Build history of the part. All positions in model axes, mm. A direction names the side the tool comes from. Give positions to 0.01 mm unless a question says otherwise; leave off trailing zeros. Loops run counter-clockwise (first coordinate to the right, second up) from the corner with the lowest first, then second, coordinate; pieces in that order, holes last.
1) 3-axis set-ups, long thin cutter, end or side, ignore diameter. For faces 5 (the cylindrical face through (50.56, -3.01, 47.15)), 6 (the flat face through (49, -97, 20)): which of +Z, -Z, +X, -X, +Y, -Y reach the whole face in a straight line?
2) Band-saw the part on C-C on y = -58.5. List the corners of the cut face in (x, z).
3) Two-plate mould, pull along X, no slides. Class faces 1 (the flat face through (49, -100, 20)), 2 (the cylindrical face through (5, -5.1, 20.3)), 3 (the flat face through (100, -49, 20)), 4 (the flat face through (49.4, -31.7, 47)): +X half, -X half, draft (parallel to the pull), parting line (faces both ways), or undercut.
4) Band-saw the part on D-D on x = 16. List the corners of the cut face in (y, z).
5) Band-saw the part on B-B on x = 50. List the corners of the cut face in (y, z).
6) Flat gauge pins, fed straight in: P1, Ø5, axis at x = 88.5, y = -24.5, coming from the -Z side; P2, Ø3, axis at x = 74.5, y = -58, coming from the -Z side. Where does each tip first touch, or does it go through?
7) Wall check: line 1 (Y direction, x = 50, z = 30); line 2 (Y direction, x = 54, z = 26); line 3 (X direction, y = -22, z = 27.5). Give the ranges that are in metal, low to high.
8) Band-saw the part on A-A on z = 23.5. List the corners of the cut face in (x, y), then the cut area to 3 significant figures.
```python
from build123d import *

# Parameters (mm, degrees)
F0_W     = 100
F0_H     = 50
F1_DEPTH = 100
F2_R     = 15
F3_DEPTH = 50
F4_R     = 10
F5_T     = -3


with BuildPart() as f1:
    # F0 (on Front) → F1 (new body)
    with BuildSketch(Plane.XZ):
        with Locations((50, 25)):
            Rectangle(F0_W, F0_H)
    extrude(amount=F1_DEPTH)

    # F2 (on face) → F3 (cut, through all)
    with BuildSketch(Plane.XY.offset(50)):
        with Locations((50, -50)):
            Circle(F2_R)
    extrude(amount=-F3_DEPTH, mode=Mode.SUBTRACT)

    # F4
    f4_edges = [f1.edges().sort_by_distance(p)[0] for p in [
        (100, 0, 25),
        (0, 0, 25),
        (100, -100, 25),
        (0, -100, 25),
        (50, -100, 50),
        (0, -50, 50),
        (100, -50, 50),
        (50, 0, 50),
    ]]
    fillet(f4_edges, radius=F4_R)

    # F5
    f5_openings = [f1.faces().sort_by_distance(p)[0] for p in [
        (1.414214, -50, 0),
    ]]
    offset(amount=F5_T, openings=f5_openings)


solid = f1.part
```
Findings below:
1. face 5: +Z, +X, -X, +Y
1. face 6: -Z
2. outline: (0, 0) - (3, 0) - (3, 40) arc R7 cw to (10, 47) - (34.13, 47) - (34.13, 0) - (37.64, 0) - (37.64, 50) - (10, 50) arc R10 ccw to (0, 40) - close; (62.36, 0) - (65.87, 0) - (65.87, 47) - (90, 47) arc R7 cw to (97, 40) - (97, 0) - (100, 0) - (100, 40) arc R10 ccw to (90, 50) - (62.36, 50) - close
3. face 1: draft
3. face 2: undercut
3. face 3: +X half
3. face 4: undercut
4. outline: (-100, 0) - (-97, 0) - (-97, 40) arc R7 cw to (-90, 47) - (-10, 47) arc R7 cw to (-3, 40) - (-3, 0) - (0, 0) - (0, 40) arc R10 ccw to (-10, 50) - (-90, 50) arc R10 ccw to (-100, 40) - close
5. outline: (-100, 0) - (-97, 0) - (-97, 40) arc R7 cw to (-90, 47) - (-68, 47) - (-68, 0) - (-65, 0) - (-65, 50) - (-90, 50) arc R10 ccw to (-100, 40) - close; (-35, 0) - (-32, 0) - (-32, 47) - (-10, 47) arc R7 cw to (-3, 40) - (-3, 0) - (0, 0) - (0, 40) arc R10 ccw to (-10, 50) - (-35, 50) - close
6. P1: stops at z = 46.93
6. P2: stops at z = 47
7. line 1: y = -100 to -97, -68 to -65, -35 to -32, -3 to 0
7. line 2: y = -100 to -97, -67.55 to -64.46, -35.54 to -32.45, -3 to 0
7. line 3: x = 0 to 3, 97 to 100
8. outline: (0, -90) arc R10 ccw to (10, -100) - (90, -100) arc R10 ccw to (100, -90) - (100, -10) arc R10 ccw to (90, 0) - (10, 0) arc R10 ccw to (0, -10) - close; circle Ø36 at (50, -50); hole (3, -90) arc R7 ccw to (10, -97) - (90, -97) arc R7 ccw to (97, -90) - (97, -10) arc R7 ccw to (90, -3) - (10, -3) arc R7 ccw to (3, -10) - close; hole circle Ø30 at (50, -50)
8. area: 1,430 mm2
